Build history of the part. All positions in model axes, mm. Face numbers are marked on the shaded views. A direction names the side the tool comes from. Round coordinates to 2 decimals unless told otherwise and drop trailing zeros. Loops run counter-clockwise (first coordinate to the right, second up) from the corner with the lowest first, then second, coordinate; pieces in that order, holes last.
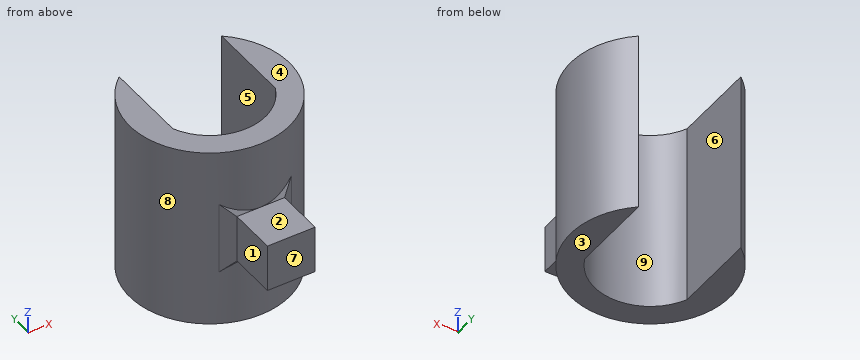
from build123d import *

# Parameters (mm, degrees)
F1_DEPTH      = 38.5
F3_W          = 10
F3_H          = 10
F4_DEPTH      = 10
F4_DEPTH_BACK = 4
F4_TAPER_BACK = -55


with BuildPart() as f1:
    # F0 (on Top) → F1 (new body)
    with BuildSketch(Plane.XY):
        with BuildLine():
            ThreePointArc((10.75, -4.7434164903), (0, -11.75), (-10.75, -4.7434164903))
            Line((-10.75, -4.7434164903), (-10.75, 12.8452325787))
            ThreePointArc((-10.75, 12.8452325787), (0, -16.75), (10.75, 12.8452325787))
            Line((10.75, 12.8452325787), (10.75, -4.7434164903))
        make_face()
    extrude(amount=F1_DEPTH)

    # F3 (on offset) → F4 (join, two sides)
    with BuildSketch(Plane.XZ.offset(16.75)) as f4_sk:
        with Locations((0, 19.25)):
            Rectangle(F3_W, F3_H)
    extrude(amount=F4_DEPTH)
    extrude(f4_sk.sketch, amount=-F4_DEPTH_BACK, taper=F4_TAPER_BACK)


solid = f1.part
(1) Slice it at C-C on x = 12. List the corners of the cut face in (y, z).
Responses:
outline: (-11.69, 0) - (11.69, 0) - (11.69, 38.5) - (-11.69, 38.5) - close
(2) Slice it at A-A on y = 0. List the corners of the cut face in (x, z).
Responses:
outline: (-16.75, 0) - (-10.75, 0) - (-10.75, 38.5) - (-16.75, 38.5) - close; (10.75, 0) - (16.75, 0) - (16.75, 38.5) - (10.75, 38.5) - close
(3) Slice it at D-D on z = 32. List the corners of the cut face in (x, y).
Responses:
outline: (-10.75, -4.74) - (-10.75, 12.85) arc R16.75 ccw (long way) to (10.75, 12.85) - (10.75, -4.74) arc R11.75 cw to start
(4) Slice it at B-B on y = -6.5. List the corners of the cut face in (x, z), plus the area to 3 significant figures.
Responses:
outline: (-15.44, 0) - (-9.79, 0) - (-9.79, 38.5) - (-15.44, 38.5) - close; (9.79, 0) - (15.44, 0) - (15.44, 38.5) - (9.79, 38.5) - close
area: 435 mm2
(5) Pin check, flat tips, straight feed: P1, Ø3, axis at y = -24, z = 17, coming from the -X side; P2, Ø8, axis at y = -17, z = 15.5, coming from the -X side; P3, Ø14, axis at y = 8.5, z = 10, coming from the -X side. Stop position of each tip, or through.
Responses:
P1: stops at x = -5
P2: stops at x = -10.56
P3: stops at x = -16.68
(6) Pull direction X, two halves, no side cores. Call the marked faces 6, 7, 8 and 9: +X half, -X half, draft (parallel to the pull), parting line (faces both ways), or undercut.
Responses:
face 6: undercut
face 7: draft
face 8: parting line
face 9: undercut
(7) Which spindle directions (+Z, -Z, +X, -X, +Y, -Y) get a long thin tool onto all of the face, cutting with end or side? Do the marked faces 1, 2, 3, 4 and 5. Say none if no direction does.
Responses:
face 1: +Z, -Z, -X, -Y
face 2: +Z, +X, -X, -Y
face 3: -Z, +X, -X, +Y, -Y
face 4: +Z, +X, -X, +Y, -Y
face 5: +Z, -Z, +Y
(8) Probe line 1 (X direction, y = -17, z = 19.5); line 2 (Z direction, x = -3.5, y = -21); line 3 (X direction, y = -3.5, z = 3.5). List the from-to ranges inside material, lowest first.
Responses:
line 1: x = -5 to 5
line 2: z = 14.25 to 24.25
line 3: x = -16.38 to -10.75, 10.75 to 16.38
